Drawing for the job (mm, zero at the part's lowest x, y, z). A direction names the side the tool comes from. Round coordinates to 2 decimals unless told otherwise and drop trailing zeros. Order: outer loops, then holes, each group sorted by start corner. A loop starts at its lowest first (then second) coordinate and runs counter-clockwise, first axis right, second up. Notation, with made-up numbers: (-37.75, 76.5) - (15.25, 76.5) arc R30 cw to (15.25, 110.5) - close; hole circle Ø11 at (70, 77.25). An arc over 180 degrees is marked (long way). Answer as a JSON object with one key per item and string values.
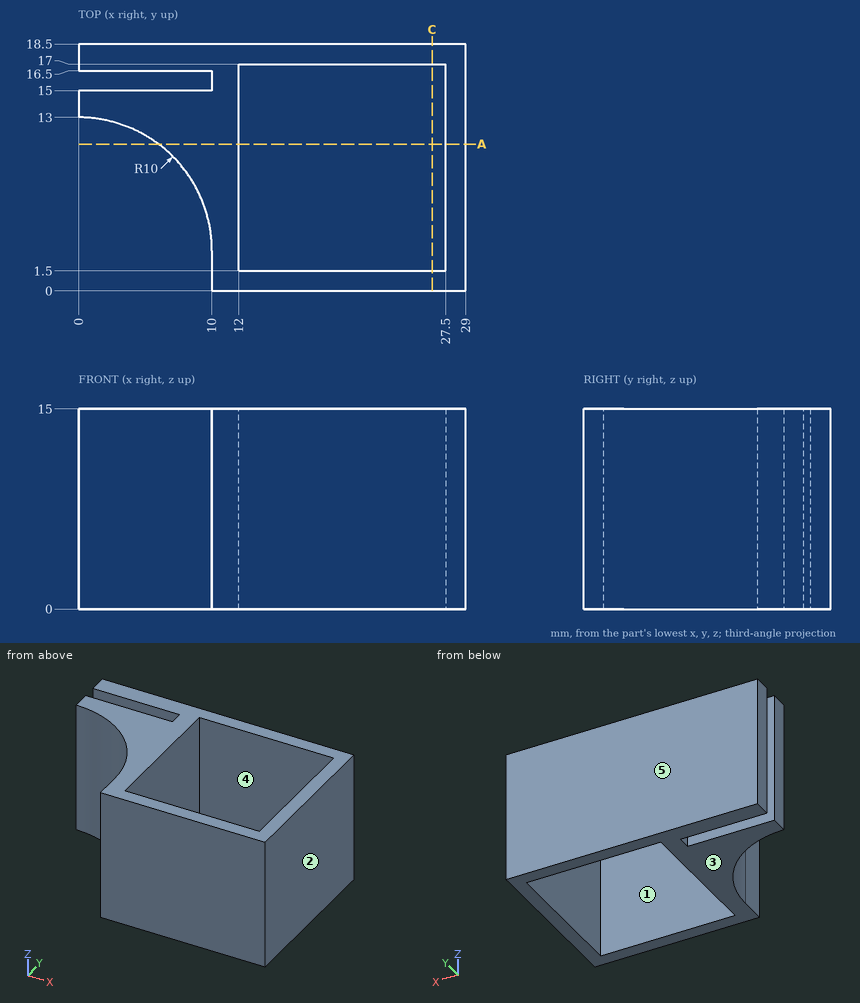
Item 1: Cut at A-A (y = 11). Write the cut outline in (x, z), plus the area to 4 significant figures.
Taken from the geometry:
{"outline": "(6, 0) - (12, 0) - (12, 15) - (6, 15) - close; (27.5, 0) - (29, 0) - (29, 15) - (27.5, 15) - close", "area": "112.5 mm2"}
Item 2: Drop flat-ended pins along their axis: P1, Ø3, axis at x = 3, z = 7, coming from the -Y side; P2, Ø5, axis at y = 6, z = 10.5, coming from the -X side; P3, Ø8, axis at x = 12.5, y = 5.5, coming from the -Z side; P4, Ø1.5, axis at y = 1.5, z = 9.5, coming from the -X side. Give the stop position or say it passes through.
Taken from the geometry:
{"P1": "y = 11.93", "P2": "x = 8.35", "P3": "z = 0", "P4": "x = 10"}
Item 3: Tool access for the marked faces 4 and 5: list every direction of +Z, -Z, +X, -X, +Y, -Y with a clear straight run to the whole face (end or side of a thin tool).
Taken from the geometry:
{"face 4": "+Z, -Z", "face 5": "+Z, -Z, +X, -X, +Y"}
Item 4: Probe L1, parallel to Y at x = 20.5, z = 10.25; L2, parallel to X at y = 16.25, z = 1; L3, parallel to X at y = 13.5, z = 6. List the from-to ranges inside material, lowest first. Write a range as from..to.
Taken from the geometry:
{"L1": "0..1.5, 17..18.5", "L2": "10..12, 27.5..29", "L3": "0..12, 27.5..29"}
Item 5: Two-plate mould, pull along X, no slides. Class the marked faces 1, 2 and 3: pulls with the +X half, pulls with the -X half, needs draft (parallel to the pull), parting line crosses it, or undercut.
Taken from the geometry:
{"face 1": "undercut", "face 2": "pulls with the +X half", "face 3": "needs draft"}
Item 6: Cut at C-C (x = 26.5). Write the cut outline in (y, z), plus the area to 3 significant figures.
Taken from the geometry:
{"outline": "(0, 0) - (1.5, 0) - (1.5, 15) - (0, 15) - close; (17, 0) - (18.5, 0) - (18.5, 15) - (17, 15) - close", "area": "45.0 mm2"}
